Check sheet for the modelled part. Datum: model origin and axes. Units: mm. Face numbers are marked on the shaded views. A direction names the side the tool comes from. Give positions to 0.01 mm unless a question says otherwise; leave off trailing zeros. Loops run counter-clockwise (first coordinate to the right, second up) from the corner with the lowest first, then second, coordinate; pieces in that order, holes last. Notation, with made-up numbers: M -3,-39 L 10,-39 A22 ccw 10,-32 Z; hole C -36.75,-33.5 d1. An arc over 180 degrees is marked long. Write each question's results on one line, items separated by ' | '. Start each with the question number.
1. Sectioned sample at D-D on x = -11.5. Record the cut outline in (y, z).
2. Tool access check on the marked faces 4 and 5. Record the directions out of +Z, -Z, +X, -X, +Y, -Y that give a thin tool (end or side, any length) a straight path to the whole face; none if there is none.
3. Sectioned sample at C-C on z = 2. Record the cut outline in (x, y).
4. Material ranges on line 1 along Y through (x, z) = (0, 2.75); line 2 along Z through (x, y) = (-13, 2.25); line 3 along X through (y, z) = (7.75, 8.5), recorded low to high.
5. Go/stop test with flat-tipped pins: pin 1 (2 mm diameter, centred on y = 2.5, z = 7.5, fed in from -X); pin 2 (2 mm diameter, centred on x = -0.5, y = 11.5, fed in from +Z); pin 3 (1.5 mm diameter, centred on x = 1.5, z = 3, fed in from -Y). Record where each tip stops, or that it passes through.
6. Sectioned sample at A-A on y = 0. Record the cut outline in (x, z).
7. Draft check along X on the marked faces 1, 2 and 3. Enter one of: pulls with the +X half, pulls with the -X half, needs draft (parallel to the pull), parting line crosses it, or undercut.
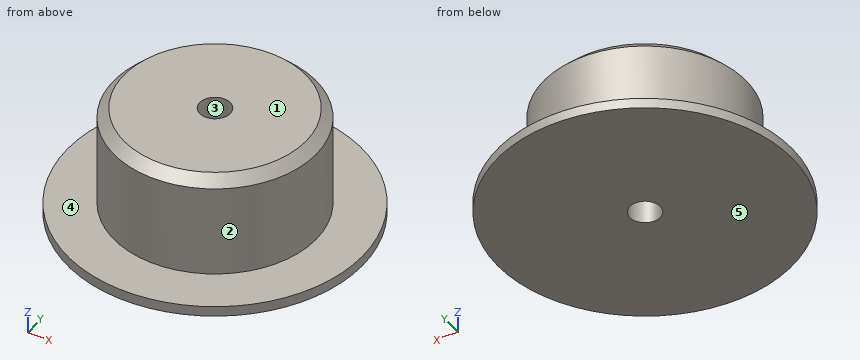
```python
from build123d import *

# Parameters (mm, degrees)
SKETCH_R      = 9.95
SKETCH_R_2    = 1.5
PAD_DEPTH     = 10
CHAMFER_SIZE  = 1
SKETCH001_R   = 14.5
SKETCH001_R_2 = 1.5
PAD001_DEPTH  = 1


with BuildPart() as part:
    # Sketch → Pad (new body)
    with BuildSketch(Plane.XY):
        Circle(SKETCH_R)
        Circle(SKETCH_R_2, mode=Mode.SUBTRACT)
    extrude(amount=PAD_DEPTH)

    # Chamfer
    chamfer_edges = [part.edges().sort_by_distance(p)[0] for p in [
        (-9.95, 0, 10),
    ]]
    chamfer(chamfer_edges, length=CHAMFER_SIZE)

    # Sketch001 (on Face3 of Chamfer) → Pad001 (join)
    with BuildSketch(Plane(origin=(0, 0, 0), x_dir=(1, 0, 0), z_dir=(0, 0, -1))):
        Circle(SKETCH001_R)
        Circle(SKETCH001_R_2, mode=Mode.SUBTRACT)
    extrude(amount=PAD001_DEPTH)


solid = part.part
```
Output values:
1) outline: M -8.83,-1 L 8.83,-1 L 8.83,0 L -8.83,0 Z
2) face 4: +Z | face 5: -Z, +X, -X, +Y, -Y
3) outline: C 0,0 d19.9; hole C 0,0 d3
4) line 1: -9.95 to -1.5, 1.5 to 9.95 | line 2: -1 to 0 | line 3: -6.24 to 6.24
5) pin 1: x = -9.84 | pin 2: z = 0 | pin 3: y = -9.92
6) outline: M -14.5,-1 L -1.5,-1 L -1.5,10 L -8.95,10 L -9.95,9 L -9.95,0 L -14.5,0 Z; M 1.5,-1 L 14.5,-1 L 14.5,0 L 9.95,0 L 9.95,9 L 8.95,10 L 1.5,10 Z
7) face 1: needs draft | face 2: parting line crosses it | face 3: undercut
